CAD build for the part. Positions are in the model's coordinates, mm. A direction names the side the tool comes from. Coordinates: 2 decimals unless noted, no trailing zeros. Loops run counter-clockwise (first coordinate to the right, second up) from the corner with the lowest first, then second, coordinate; pieces in that order, holes last. Notation, with made-up numbers: (34.5, 50) -> (55.5, 50) arc R25 cw to (55.5, 89) -> close; hole circle Ø5 at (-36, 56.25). An arc over 180 degrees is marked (long way). Write each question's results on one line, items separated by ' | '.
```python
from build123d import *

# Parameters (mm, degrees)
EXTRUDE1_DEPTH     = 5
CUT_EXTRUDE1_DEPTH = 3
SKETCH1_W          = 36.36
SKETCH1_H          = 33.2
SKETCH1_W_2        = 34.36
SKETCH1_H_2        = 31.2
CUT_EXTRUDE2_DEPTH = 0.1


with BuildPart() as part:
    # COMPONENT_OUTLINE → Extrude1 (new body)
    with BuildSketch(Plane.XY):
        Polygon((19.18, -24.5), (20.18, -24.5), (20.18, -14.5), (19.18, -14.5), (19.18, 1.25), (-19.18, 1.25), (-19.18, -33.95), (19.18, -33.95), align=None)
    extrude(amount=EXTRUDE1_DEPTH)

    # Sketch2 → Cut-Extrude1 (cut)
    with BuildSketch(Plane(origin=(0, 0, 0), x_dir=(-1, 0, 0), z_dir=(0, 0, -1))):
        Polygon((-19.18, -24.5), (-19.18, -33.95), (19.18, -33.95), (19.18, 1.25), (-19.18, 1.25), (-19.18, -14.5), (-20.18, -14.5), (-20.18, -24.5), align=None)
        Polygon((-16.18, -21.5), (-16.18, -30.95), (16.18, -30.95), (16.18, -1.75), (-16.18, -1.75), (-16.18, -17.5), (-17.18, -17.5), (-17.18, -21.5), align=None, mode=Mode.SUBTRACT)
    extrude(amount=-CUT_EXTRUDE1_DEPTH, mode=Mode.SUBTRACT)

    # Sketch1 → Cut-Extrude2 (cut)
    with BuildSketch(Plane.XY.offset(5)):
        with Locations((0, -16.35)):
            Rectangle(SKETCH1_W, SKETCH1_H)
        with Locations((0, -16.35)):
            Rectangle(SKETCH1_W_2, SKETCH1_H_2, mode=Mode.SUBTRACT)
    extrude(amount=-CUT_EXTRUDE2_DEPTH, mode=Mode.SUBTRACT)


solid = part.part
```
Q1. Wall check: L1, parallel to X at y = -3.5, z = 4.3; L2, parallel to Y at x = 15, z = 1.6; L3, parallel to X at y = -10, z = 1.6. Give the ranges that are in metal, low to high. Write a range as from..to.
Results are:
L1: -19.18..19.18 | L2: -30.95..-1.75 | L3: -16.18..16.18
Q2. Cut at B-B on y = -17. Write the cut outline in (x, z).
Results are:
outline: (-19.18, 3) -> (-16.18, 3) -> (-16.18, 0) -> (16.18, 0) -> (16.18, 3) -> (20.18, 3) -> (20.18, 5) -> (18.18, 5) -> (18.18, 4.9) -> (17.18, 4.9) -> (17.18, 5) -> (-17.18, 5) -> (-17.18, 4.9) -> (-18.18, 4.9) -> (-18.18, 5) -> (-19.18, 5) -> close
Q3. Drop flat-ended pins along their axis: pin 1 (2.5 mm diameter, centred on y = -20, z = 1, fed in from -X); pin 2 (3 mm diameter, centred on x = 6.5, z = 1, fed in from +Y); pin 3 (0.8 mm diameter, centred on x = 16.5, z = 2, fed in from -Y). Give the stop position or say it passes through.
Results are:
pin 1: x = -16.18 | pin 2: y = -1.75 | pin 3: y = -30.95
Q4. Cut at C-C on x = 3. Write the cut outline in (y, z), and give its area (3 significant figures).
Results are:
outline: (-33.95, 3) -> (-30.95, 3) -> (-30.95, 0) -> (-1.75, 0) -> (-1.75, 3) -> (1.25, 3) -> (1.25, 5) -> (0.25, 5) -> (0.25, 4.9) -> (-0.75, 4.9) -> (-0.75, 5) -> (-31.95, 5) -> (-31.95, 4.9) -> (-32.95, 4.9) -> (-32.95, 5) -> (-33.95, 5) -> close | area: 158 mm^2
Q5. Cut at A-A on z = 4. Write the cut outline in (x, y).
Results are:
outline: (-19.18, -33.95) -> (19.18, -33.95) -> (19.18, -24.5) -> (20.18, -24.5) -> (20.18, -14.5) -> (19.18, -14.5) -> (19.18, 1.25) -> (-19.18, 1.25) -> close
Q6. Which spindle directions (+Z, -Z, +X, -X, +Y, -Y) get a long thin tool onto all of the face, cutting with end or side? Do faces 1 (the flat face through (0, -1.75, 1)), 2 (the flat face through (-16.18, -17, 1)), 3 (the flat face through (17.18, -19, 1)). Say none if no direction does.
Results are:
face 1: -Z, +X, -X, +Y | face 2: -Z, -X, +Y, -Y | face 3: -Z, +X, +Y, -Y
